Can you work these out from the model? Positions are in its coordinate system, mm. A direction names the side the tool comes from. Give positions to 0.01 mm unless a question says otherwise; leave off trailing zeros. Order: outer loops, then holes, each group sorted by start corner. A loop starts at its lowest first (then second) coordinate and runs counter-clockwise, first axis right, second up. Notation, with made-up numbers: (34, -33.5) -> (59, -33.5) arc R13 ccw to (59, -29.5) -> close; hole circle Ø11 at (56.25, 14.25). An arc over 180 degrees is marked (long way). Answer as a JSON object with one key per item and string values.
```python
from build123d import *

# Parameters (mm, degrees)
SKETCH_1_W          = 860
SKETCH_1_H          = 100
SKETCH_1_R          = 13
EXTRUDE_1_DEPTH     = 8
SKETCH_2_W          = 860
SKETCH_2_H          = 8
EXTRUDE_2_DEPTH     = 92
CUT_EXTRUDE_1_DEPTH = 453.65881191


with BuildPart() as part:
    # 草图1 → 凸台-拉伸1 (new body)
    with BuildSketch(Plane.XY):
        with Locations((0, 50)):
            Rectangle(SKETCH_1_W, SKETCH_1_H)
        with Locations((390, 40)):
            Circle(SKETCH_1_R, mode=Mode.SUBTRACT)
        with Locations((310, 40)):
            Circle(SKETCH_1_R, mode=Mode.SUBTRACT)
        with Locations(Location((-390, 40, 0), (0, 0, 180))):
            Circle(SKETCH_1_R, mode=Mode.SUBTRACT)
        with Locations(Location((-310, 40, 0), (0, 0, 180))):
            Circle(SKETCH_1_R, mode=Mode.SUBTRACT)
    extrude(amount=EXTRUDE_1_DEPTH)

    # 草图2 → 凸台-拉伸2 (add)
    with BuildSketch(Plane.XY.offset(8)):
        with Locations((0, 96)):
            Rectangle(SKETCH_2_W, SKETCH_2_H)
    extrude(amount=EXTRUDE_2_DEPTH)

    # 草图4 → 切除-拉伸1 (cut, through all)
    with BuildSketch(Plane(origin=(0, 100, 0), x_dir=(1, 0, 0), z_dir=(0, 1, 0))):
        Polygon((-430, -15), (-390, -15), (-305, -100), (-430, -100), align=None)
    cut_extrude_1 = extrude(amount=-CUT_EXTRUDE_1_DEPTH, mode=Mode.SUBTRACT)

    # 镜向1: 切除-拉伸1 across plane
    add(cut_extrude_1.mirror(Plane(origin=(0, 0, 0), x_dir=(0, 0, 1), z_dir=(1, 0, 0))), mode=Mode.SUBTRACT)


solid = part.part
```
1. If we section it at A-A on y = 40: Please give me the cut outline in (x, z).
Worked answers:
{"outline": "(-430, 0) -> (-403, 0) -> (-403, 8) -> (-430, 8) -> close; (-377, 0) -> (-323, 0) -> (-323, 8) -> (-377, 8) -> close; (-297, 0) -> (297, 0) -> (297, 8) -> (-297, 8) -> close; (323, 0) -> (377, 0) -> (377, 8) -> (323, 8) -> close; (403, 0) -> (430, 0) -> (430, 8) -> (403, 8) -> close"}
2. If we mould it in two halves opening along X, with no side actions, what happens to faces 3 (the face through (-297.013, 39.428, 3.944)), 4 (the face through (-6, 92, 53)), 5 (the face through (348, 96, 57))? For each: +X half, -X half, draft (parallel to the pull), parting line (faces both ways), or undercut.
Worked answers:
{"face 3": "undercut", "face 4": "draft", "face 5": "+X half"}
3. If we section it at B-B on x = 339: Please give me the cut outline in (y, z).
Worked answers:
{"outline": "(0, 0) -> (100, 0) -> (100, 66) -> (92, 66) -> (92, 8) -> (0, 8) -> close"}
4. If we section it at D-D on z = 23: Please give me the cut outline in (x, y).
Worked answers:
{"outline": "(-382, 92) -> (382, 92) -> (382, 100) -> (-382, 100) -> close"}
5. Will these pins go through, and if not, where does the flat tip stop? pin 1 Ø2.5 at (x, y) = (-418, 94.5) entering from +Z; pin 2 Ø5 at (x, z) = (116.5, 39.5) entering from -Y; pin 3 Ø3 at (x, y) = (-198, 77.5) entering from +Z.
Worked answers:
{"pin 1": "z = 15", "pin 2": "y = 92", "pin 3": "z = 8"}
6. If we section it at C-C on z = 59: Please give me the cut outline in (x, y), then the cut area to 3 significant figures.
Worked answers:
{"outline": "(-346, 92) -> (346, 92) -> (346, 100) -> (-346, 100) -> close", "area": "5,540 mm²"}
7. For faces 1 (the face through (-430, 49, 4)), 2 (the face through (-6, 47, 8)), which set-ups out of +Z, -Z, +X, -X, +Y, -Y let a thin tool reach every point of the face, with its end or its side?
Worked answers:
{"face 1": "+Z, -Z, -X, +Y, -Y", "face 2": "+Z, +X, -X, -Y"}
8. Please list where these lines run through material, in increasing order: L1, parallel to Y at x = 310, z = 2; L2, parallel to Z at x = 377, y = 25; L3, parallel to Y at x = -77, z = 37.
Worked answers:
{"L1": "0 to 27, 53 to 100", "L2": "0 to 8", "L3": "92 to 100"}
